Could you check a few things on this drawing? It's one solid part, dimensions in mm from its lowest x, y, z. A direction names the side the tool comes from. Round coordinates to 2 decimals unless told otherwise and drop trailing zeros. Order: outer loops, then holes, each group sorted by start corner. A loop starts at its lowest first (then second) coordinate and runs counter-clockwise, first axis right, second up.
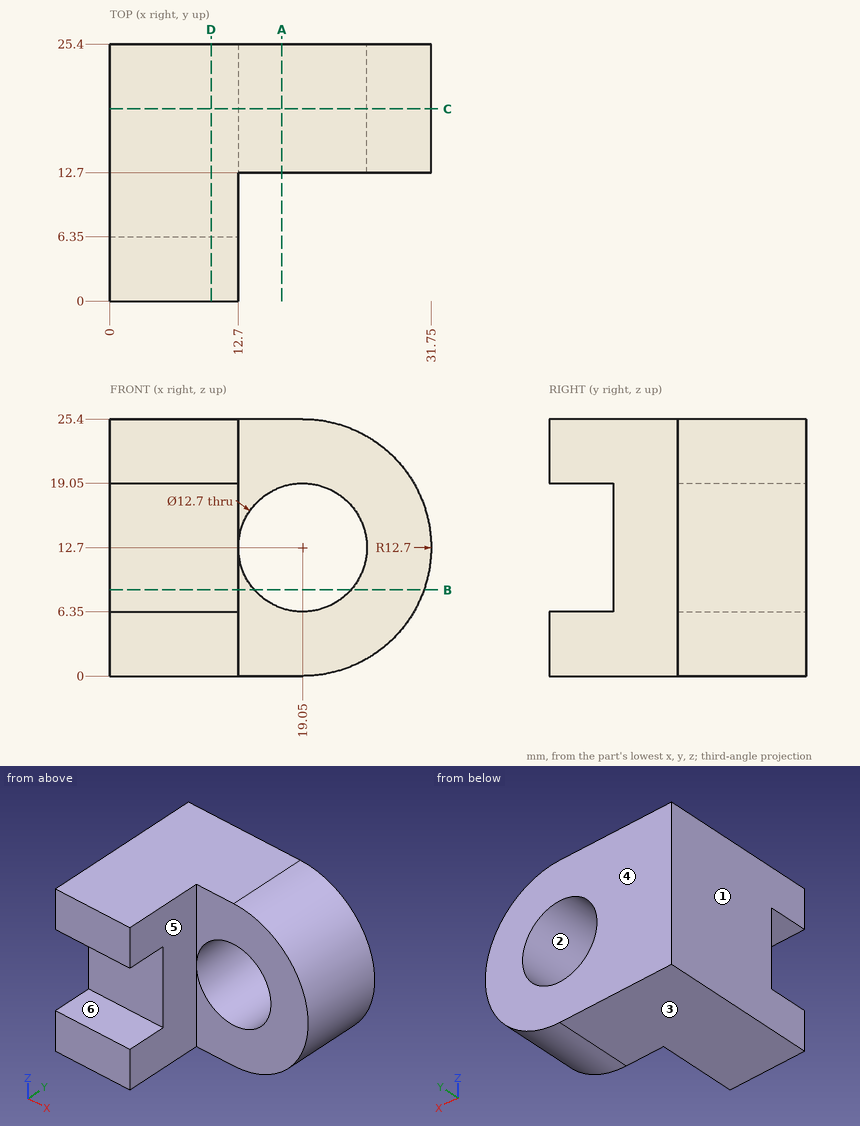
(1) If we mould it in two halves opening along Z, with no side actions, what happens to the marked faces 1, 2 and 3? For each: pulls with the +Z half, pulls with the -Z half, needs draft (parallel to the pull), parting line crosses it, or undercut.
(2) On a 3-axis mill with a long thin cutter (end or side, diameter ignored), from which of +Z, -Z, +X, -X, +Y, -Y can I reach the whole of each face in a straight line? I mean the marked faces 4, 5 and 6. Say none if no direction works.
(3) I want a section at C-C, the plane y = 19. List the corners of the cut face in (x, z) for me, plus the area to 3 significant figures.
(4) I want a section at A-A, the plane x = 17. List the corners of the cut face in (y, z) for me, plus the area to 3 significant figures.
(5) I want a section at B-B, the plane z = 8.5. List the corners of the cut face in (x, y) for me.
(6) I want a section at D-D, the plane x = 10. List the corners of the cut face in (y, z) for me, plus the area to 3 significant figures.
(7) I'm going to push flat-ended pins straight in: pin 1 Ø2 at (y, z) = (17, 18.5) entering from +X; pin 2 Ø1 at (x, y) = (23.5, 20.5) entering from +Z; pin 3 Ø12 at (x, z) = (24, 15.5) entering from -Y. Where does each tip first touch, or does it pass through?
(8) Please list where these lines run through material, in increasing order: probe 1 along Z at (x, y) = (19.05, 19.5); probe 2 along Y at (x, z) = (19, 3).
Ans:
1. face 1: needs draft
1. face 2: undercut
1. face 3: pulls with the -Z half
2. face 4: +Z, -Z, +X, -X, +Y
2. face 5: +Z, -Z, +X, -Y
2. face 6: +X, -X, -Y
3. outline: (0, 0) - (19.05, 0) arc R12.7 ccw to (19.05, 25.4) - (0, 25.4) - close; hole circle Ø12.7 at (19.05, 12.7)
3. area: 611 mm2
4. outline: (12.7, 0) - (25.4, 0) - (25.4, 6.69) - (12.7, 6.69) - close; (12.7, 18.71) - (25.4, 18.71) - (25.4, 25.4) - (12.7, 25.4) - close
4. area: 170 mm2
5. outline: (0, 6.35) - (12.7, 6.35) - (12.7, 12.7) - (14.29, 12.7) - (14.29, 25.4) - (0, 25.4) - close; (23.81, 12.7) - (31.04, 12.7) - (31.04, 25.4) - (23.81, 25.4) - close
6. outline: (0, 0) - (25.4, 0) - (25.4, 25.4) - (0, 25.4) - (0, 19.05) - (6.35, 19.05) - (6.35, 6.35) - (0, 6.35) - close
6. area: 565 mm2
7. pin 1: stops at x = 30.81
7. pin 2: stops at z = 24.77
7. pin 3: stops at y = 12.7
8. probe 1: z = 0 to 6.35, 19.05 to 25.4
8. probe 2: y = 12.7 to 25.4
